Build history of the part. All positions in model axes, mm. Round coordinates to 2 decimals unless told otherwise and drop trailing zeros. Write each loop counter-clockwise with the first axis right and the second up, starting at its lowest first coordinate (ties: lowest second). Pieces come first, ordered by that corner, then holes. Notation, with made-up numbers: M 79.25,-1 L 104.25,-1 A13 ccw 104.25,21 Z; hole C 23.5,-14.5 d2. An arc over 180 degrees is marked long. Write item = value, one per line.
Autodesk Inventor part; units mm, degrees
ref_plane "YZ Plane" through (0, 0, 0) normal (1, 0, 0) x (0, 1, 0)
ref_plane "XZ Plane" through (0, 0, 0) normal (0, 1, 0) x (-1, 0, 0)
ref_plane "XY Plane" through (0, 0, 0) normal (0, 0, 1) x (1, 0, 0)
sketch "Эскиз1" plane through (0, 0, 0) normal (0, 1, 0) x (-1, 0, 0)
  line L0 (118.7568, 10.0335) -> (3.7568, 10.0335)
  line L1 (-3.7432, 2.5335) -> (-3.7432, -10.4665)
  line L2 (-3.7432, -10.4665) -> (126.2568, -10.4665)
  line L3 (126.2568, -10.4665) -> (126.2568, 2.5335)
  arc A0 (3.7568, 10.0335) -> (-3.7432, 2.5335) centre (3.7568, 2.5335) ccw
  arc A1 (126.2568, 2.5335) -> (118.7568, 10.0335) centre (118.7568, 2.5335) ccw
  point P0 (0, 0)
  point P1 (-3.7432, 10.0335)
  dimension "d0" = 20.5
  dimension "d1" = 130
  dimension "d2" = 7.5
  dimension "d3" = 7.5
extrude "Выдавливание1" add sketch "Эскиз1" along normal blind 1.5
sketch "Эскиз2" plane through (0, 1.5, 0) normal (0, 1, 0) x (1, 0, 0)
  line L0 (3.7432, -2.5335) -> (3.7432, 10.4665)
  line L1 (-126.2568, 10.4665) -> (-126.2568, -2.5335)
  line L2 (3.7432, 10.4665) -> (-126.2568, 10.4665)
  line L3 (-126.2568, 10.4665) -> (-126.2568, 8.4665)
  line L4 (-126.2568, 8.4665) -> (3.7432, 8.4665)
  line L5 (3.7432, 8.4665) -> (3.7432, 10.4665)
  point P0 (0, 0)
  point P1 (3.7432, 8.4665)
  dimension "d6" = 2
extrude "Выдавливание2" add sketch "Эскиз2" along normal blind 8.2
fillet "Сопряжение1" radius 4.5 1 edges at (3.7432, 9.7, -9.4665)
fillet "Сопряжение2" radius 4.5 1 edges at (-126.2568, 9.7, -9.4665)
sketch "Эскиз3" plane through (-126.2568, 1.5, -8.4665) normal (0, 0, 1) x (1, 0, 0)
  line L0 (125.5, 8.2) -> (4.5, 8.2)
  line L1 (117, 8.2) -> (121.5, 8.2)
  line L2 (121.5, 8.2) -> (121.5, 6.95)
  line L3 (121.5, 6.95) -> (117, 6.95)
  line L4 (117, 6.95) -> (117, 8.2)
  line L5 (130, 0) -> (130, 3.7)
  line L6 (63, 8.2) -> (67.5, 8.2)
  line L7 (67.5, 8.2) -> (67.5, 6.95)
  line L8 (67.5, 6.95) -> (63, 6.95)
  line L9 (63, 6.95) -> (63, 8.2)
  line L10 (5, 8.2) -> (8.5, 8.2)
  line L11 (8.5, 8.2) -> (8.5, 6.95)
  line L12 (8.5, 6.95) -> (5, 6.95)
  line L13 (5, 6.95) -> (5, 8.2)
  point P0 (126.2568, -1.5)
  point P1 (121.5, 7.575)
  point P2 (63, 7.575)
  point P3 (67.5, 7.575)
  point P4 (8.5, 8.2)
  dimension "d11" = 8.5
  dimension "d12" = 4.5
  dimension "d13" = 1.25
  dimension "d14" = 58.5
  dimension "d15" = 4.5
  dimension "d16" = 1.25
  dimension "d17" = 62.5
  dimension "d18" = 3.5
  dimension "d19" = 1.25
extrude "Выдавливание3" add sketch "Эскиз3" along normal blind 1.65
ref_plane "РабПлоскость1" through (-13.7568, 0, 2.5335) normal (1, 0, 0) x (0, 0, -1)
sketch "Эскиз4" plane through (-13.7568, 0, 2.5335) normal (1, 0, 0) x (0, 0, -1)
  line L0 (-9.5515, 3.8793) -> (-9.5515, 2.1493)
  line L1 (-9.5515, 3.8793) -> (-7.6452, 3.758)
  line L2 (-6.0216, 2.729) -> (-5.3427, 1.5)
  line L3 (-7.5, 1.5) -> (-7.5, 3.23)
  arc A0 (-6.0216, 2.729) -> (-7.6452, 3.758) centre (-7.7722, 1.762) ccw
  line L4 (-8.5983, 0.5037) -> (-8.5983, 3.23) construction
  line L5 (-9.6967, 1.602) -> (-9.6967, 2.1317)
  line L6 (-7.5, 2.1317) -> (-7.5, 1.602)
  arc A1 (-9.6967, 1.602) -> (-7.5, 1.602) centre (-8.5983, 1.602) ccw
  arc A2 (-7.5, 2.1317) -> (-9.6967, 2.1317) centre (-8.5983, 2.1317) ccw
  line L7 (0, 1.5) -> (-7.5, 1.5)
  line L8 (-5.3427, 1.5) -> (-7.5, 1.5)
  point P0 (2.5335, 0)
  point P1 (-6.5515, 3.6883)
  point P2 (-8.5983, 1.8668)
  point P3 (-9.5515, 2.6775)
  dimension "d23" = 1.73
  dimension "d24" = 3
  dimension "d25" = 2.5
  dimension "d26" = 1.73
  dimension "d27" = 2
extrude "Выдавливание4" add sketch "Эскиз4" along normal blind 5 contours L1 A0 L2 L7 L3 A2 L0
ref_plane "РабПлоскость2" through (-40.7568, 0, 2.5335) normal (1, 0, 0) x (0, 0, -1)
mirror "Зеркальное отражение1" about plane through (-40.7568, 0, 2.5335) normal (1, 0, 0) of "Выдавливание4"
ref_plane "РабПлоскость3" through (-60.7568, 0, 2.5335) normal (1, 0, 0) x (0, 0, -1)
mirror "Зеркальное отражение2" about plane through (-60.7568, 0, 2.5335) normal (1, 0, 0) of "Выдавливание4"
sketch "Эскиз5" plane through (0, 1.5, 0) normal (0, 1, 0) x (1, 0, 0)
  point P0 (0, 0)
ref_plane "РабПлоскость4" through (0, 6, 0) normal (0, 1, 0) x (1, 0, 0)
sketch "Эскиз6" plane through (0, 6, 0) normal (0, 1, 0) x (1, 0, 0)
  line L0 (-107.513, 6.4665) -> (-116.163, 6.4665)
  line L1 (-116.163, 6.4665) -> (-116.163, -5.5335)
  line L2 (-116.163, -5.5335) -> (-107.513, -5.5335)
  line L3 (-107.513, -5.5335) -> (-107.513, 6.4665)
  line L4 (-117.7568, 8.4665) -> (-63.2568, 8.4665)
  point P0 (0, 0)
  point P1 (-111.838, 6.4665)
  dimension "d33" = 12
  dimension "d34" = 8.65
  dimension "d35" = 2
properties part number "k400+ крышка"
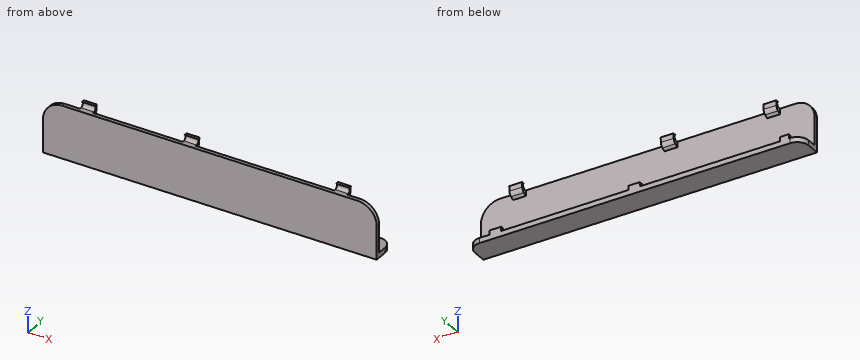
1. Band-saw the part on C-C (x = -81). List the corners of the cut face in (y, z), plus the area to 4 significant figures.
Responses:
outline = M 0,-10.47 L 9.7,-10.47 L 9.7,-8.47 L 1.5,-8.47 L 1.5,10.03 L 0,10.03 Z
area = 47.15 mm²
2. Band-saw the part on B-B (z = -0.5). List the corners of the cut face in (x, y), plus the area to 3 significant figures.
Responses:
outline = M -126.26,0 L 3.74,0 L 3.74,1.5 L -126.26,1.5 Z
area = 195 mm²
3. Flat gauge pins, fed straight in: pin 1 (0.6 mm diameter, centred on x = -64, y = 1, fed in from +Z); pin 2 (8 mm diameter, centred on x = -19, z = 9, fed in from +Y); pin 3 (2.5 mm diameter, centred on y = 3, z = 9, fed in from +X); pin 4 (1.8 mm diameter, centred on x = -120, z = -8, fed in from -Y). Where does each tip first touch, or does it go through?
Responses:
pin_1 = 10.03
pin_2 = 1.5
pin_3 = -8.76
pin_4 = 0
4. Band-saw the part on A-A (x = -60.5). List the corners of the cut face in (y, z).
Responses:
outline = M 0,-10.47 L 9.7,-10.47 L 9.7,-6.82 L 8.45,-6.82 L 8.45,-8.47 L 1.5,-8.47 L 1.5,10.03 L 0,10.03 Z
5. Probe probe 1 along Y at (x, z) = (-121, 7.25); probe 2 along Z at (x, y) = (-79, 3.5); probe 3 along Z at (x, y) = (-76.5, 1). List the from-to ranges inside material, lowest first.
Responses:
probe_1 = 0 to 1.5
probe_2 = -10.47 to -8.47
probe_3 = -10.47 to 10.03
6. Band-saw the part on D-D (y = 7). List the corners of the cut face in (x, z), plus the area to 3 significant figures.
Responses:
outline = M -125.88,-10.47 L 3.37,-10.47 L 3.37,-8.47 L -125.88,-8.47 Z
area = 258 mm²
